Part model, mm, in its own coordinate system. A direction names the side the tool comes from. Round coordinates to 2 decimals unless told otherwise and drop trailing zeros. Order: outer loops, then holes, each group sorted by start corner. A loop starts at its lowest first (then second) coordinate and runs counter-clockwise, first axis right, second up. Notation, with made-up numbers: (20.25, 67) -> (64.25, 67) arc R25 cw to (64.25, 95) -> close; hole circle Ø2 at (65.5, -1). An arc over 180 degrees is marked (long way). Return JSON: item names as keys, results as strings. Group by question number.
from build123d import *

# Parameters (mm, degrees)
F0_R     = 11.5
F1_DEPTH = 10.5
F2_R     = 8
F3_DEPTH = 35
F4_R     = 11.5
F5_DEPTH = 4.5


with BuildPart() as f1:
    # F0 (on Top) → F1 (new body)
    with BuildSketch(Plane.XY):
        Circle(F0_R)
    extrude(amount=F1_DEPTH)

    # F2 (on face) → F3 (join)
    with BuildSketch(Plane(origin=(0, 0, 0), x_dir=(1, 0, 0), z_dir=(0, 0, -1))):
        Circle(F2_R)
    extrude(amount=F3_DEPTH)

    # F4 (on face) → F5 (cut)
    with BuildSketch(Plane.XY.offset(10.5)):
        Circle(F4_R)
        with BuildLine():
            ThreePointArc((0.575, 7), (7.575, 0), (0.575, -7))
            Line((0.575, -7), (-0.575, -7))
            ThreePointArc((-0.575, -7), (-7.575, 0), (-0.575, 7))
            Line((-0.575, 7), (0.575, 7))
        make_face(mode=Mode.SUBTRACT)
    extrude(amount=-F5_DEPTH, mode=Mode.SUBTRACT)


solid = f1.part
(1) Saw through at A-A, the plane y = 0. List the corners of the cut face in (x, z) (3 decimals).
(2) Saw through at C-C, the plane z = -3. List the corners of the cut face in (x, y).
(3) Probe L1, parallel to Z at x = 5.25, y = 6.5; L2, parallel to X at y = -5, z = -20.5 (3 decimals); L3, parallel to Y at x = -2.5, z = 5. List the from-to ranges inside material, lowest first. Write a range as [from, to].
(4) Saw through at D-D, the plane y = 8.75. List the corners of the cut face in (x, z), and give its area (3 significant figures).
(5) Saw through at B-B, the plane x = 0. List the corners of the cut face in (y, z), and give its area (3 significant figures).
(6) Pin check, flat tips, straight feed: P1, Ø5, axis at y = -9, z = -30, coming from the -X side; P2, Ø8, axis at x = 8.5, y = 8.5, coming from the +Z side; P3, Ø10, axis at x = -8, y = 1.5, coming from the -Z side; P4, Ø8, axis at x = 7, z = -14, coming from the +Y side. Stop position of each tip, or through.
(7) Tool access for faces 1 (the cylindrical face through (-1.73, 7.81, -17.26)), 2 (the flat face through (0, 7, 8)), 3 (the flat face through (0, -7, 8)): list every direction of +Z, -Z, +X, -X, +Y, -Y with a clear straight run to the whole face (end or side of a thin tool).
Results are:
{
 "1": {"outline": "(-11.5, 0) -> (-8, 0) -> (-8, -35) -> (8, -35) -> (8, 0) -> (11.5, 0) -> (11.5, 6) -> (7.575, 6) -> (7.575, 10.5) -> (-7.575, 10.5) -> (-7.575, 6) -> (-11.5, 6) -> close"},
 "2": {"outline": "circle Ø16 at (0, 0)"},
 "3": {"L1": "z = [0, 6]", "L2": "x = [-6.245, 6.245]", "L3": "y = [-11.22, 11.22]"},
 "4": {"outline": "(-7.46, 0) -> (7.46, 0) -> (7.46, 6) -> (-7.46, 6) -> close", "area": "89.5 mm^2"},
 "5": {"outline": "(-11.5, 0) -> (-8, 0) -> (-8, -35) -> (8, -35) -> (8, 0) -> (11.5, 0) -> (11.5, 6) -> (7, 6) -> (7, 10.5) -> (-7, 10.5) -> (-7, 6) -> (-11.5, 6) -> close", "area": "761 mm^2"},
 "6": {"P1": "stops at x = -4.66", "P2": "stops at z = 6", "P3": "stops at z = -35", "P4": "stops at y = 7.42"},
 "7": {"face 1": "-Z", "face 2": "+Z, +X, -X, +Y", "face 3": "+Z, +X, -X, -Y"}
}
